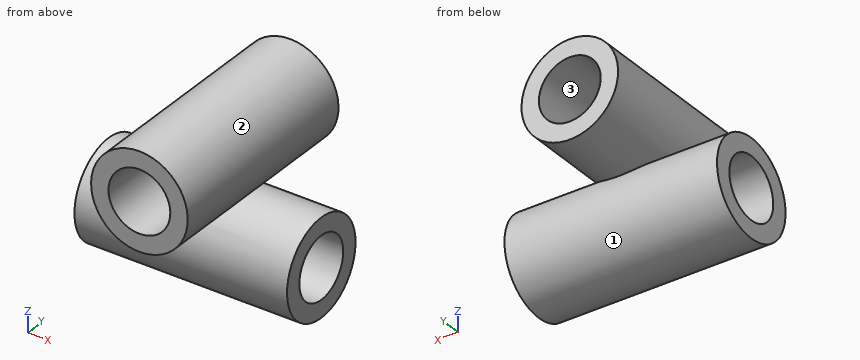
from build123d import *

# Parameters (mm, degrees)
SKETCH2_R                = 25
SKETCH2_R_2              = 16
BOSS_EXTRUDE1_DEPTH      = 110
BOSS_EXTRUDE3_DEPTH      = 55
BOSS_EXTRUDE3_DEPTH_BACK = 55
SKETCH3_R                = 25
SKETCH5_R                = 16
CUT_EXTRUDE2_DEPTH       = 110


with BuildPart() as part:
    # Sketch2 → Boss-Extrude1 (new body)
    with BuildSketch(Plane(origin=(0, 0, 0), x_dir=(1, 0, 0), z_dir=(0, 1, 0))):
        with Locations(Location((0, 0, 0), (0, 0, 270))):
            Circle(SKETCH2_R)
        with Locations(Location((0, 0, 0), (0, 0, 270))):
            Circle(SKETCH2_R_2, mode=Mode.SUBTRACT)
    extrude(amount=BOSS_EXTRUDE1_DEPTH)

    # Sketch3 → Boss-Extrude3 (add, two sides: drawn at the far end of the back side and taken through both)
    with BuildSketch(Plane(origin=(0, 0, 0), x_dir=(0, 0, -1), z_dir=(1, 0, 0)).offset(-BOSS_EXTRUDE3_DEPTH_BACK)):
        with Locations((41.031680292, 55.145345171)):
            Circle(SKETCH3_R)
    extrude(amount=BOSS_EXTRUDE3_DEPTH + BOSS_EXTRUDE3_DEPTH_BACK)

    # Sketch5 → Cut-Extrude2 (cut)
    with BuildSketch(Plane(origin=(55, 0, 0), x_dir=(0, 0, -1), z_dir=(1, 0, 0))):
        with Locations((41.031680292, 55.145345171)):
            Circle(SKETCH5_R)
    extrude(amount=-CUT_EXTRUDE2_DEPTH, mode=Mode.SUBTRACT)


solid = part.part
Verification items for the finished model (mm, model axes). Face numbers are marked on the shaded views. Coordinates: 2 decimals unless noted, no trailing zeros. Order: outer loops, then holes, each group sorted by start corner. A loop starts at its lowest first (then second) coordinate and runs counter-clockwise, first axis right, second up. Notation, with made-up numbers: M 40.25,12 L 87.25,12 A18 ccw 87.25,40 Z; hole C -14.5,26.5 d11. An arc over 180 degrees is marked long. One line per item, written item: value. Start each with the question number.
Item 1: Mould release check, pull along X, two halves, no side actions. Record for the marked faces 1, 2 and 3: released by +X, released by -X, zero draft, split by the parting line, or undercut.
Item 2: Sectioned sample at B-B (z = 0). Enter the section's corners in (x, y).
Item 3: Sectioned sample at D-D (y = 92.5). Enter the section's corners in (x, z), then the cut area to 3 significant figures.
Item 4: Gauge pin test, flat ends, axial feed: pin 1 (2 mm diameter, centred on x = 20, y = 78, fed in from +Z); pin 2 (5 mm diameter, centred on x = 14.5, y = 61, fed in from +Z); pin 3 (3 mm diameter, centred on x = 0, z = -32, fed in from +Y). Record the tip position at first contact, or that the pin passes through.
Item 5: Sectioned sample at A-A (x = -5.5). Enter the section's corners in (y, z).
Item 6: Scan lines: probe 1 along X at (y, z) = (50, 0); probe 2 along Z at (x, y) = (-11, 41) (3 decimals); probe 3 along Y at (x, z) = (-26, -55). Record each from-to range of solid material in increasing order.
Item 7: Sectioned sample at C-C (y = 62). Enter the section's corners in (x, z).
Conclusion:
1. face 1: zero draft
1. face 2: split by the parting line
1. face 3: undercut
2. outline: M -25,0 L -16,0 L -16,110 L -25,110 Z; M 16,0 L 25,0 L 25,110 L 16,110 Z
3. outline: C 0,0 d50; hole C 0,0 d32
3. area: 1,160 mm^2
4. pin 1: stops at z = 16.25
4. pin 2: stops at z = 21.93
4. pin 3: stops at y = 78.98
5. outline: M 0,-24.39 L 36.49,-24.39 A25 ccw long 73.8,-24.39 L 110,-24.39 L 110,-15.02 L 0,-15.02 Z; M 0,15.02 L 110,15.02 L 110,24.39 L 0,24.39 Z; hole C 55.15,-41.03 d32
6. probe 1: x = -25 to -16, 16 to 25
6. probe 2: z = -61.645 to -48.509, -33.554 to -11.619, 11.619 to 22.45
6. probe 3: y = 34.41 to 47.34, 62.95 to 75.88
7. outline: M -55,-65.07 L 55,-65.07 L 55,-55.49 L -55,-55.49 Z; M -55,-26.57 L 55,-26.57 L 55,-16.99 L 18.34,-16.99 A25 ccw long -18.34,-16.99 L -55,-16.99 Z; hole C 0,0 d32
